Could you check a few things on this drawing? It's one solid part, dimensions in mm from its lowest x, y, z. A direction names the side the tool comes from. Give positions to 0.01 mm unless a question says otherwise; leave off trailing zeros. Loops run counter-clockwise (first coordinate to the right, second up) from the corner with the lowest first, then second, coordinate; pieces in that order, holes last.
1. I need wall thicknesses on line 1 along Y through (x, z) = (6, 24.25); line 2 along X through (y, z) = (3.25, 16.5) (1 decimal); line 3 along Z through (x, y) = (35.5, 8.75). Which ranges of each line are inside material? Lowest first, please.
2. Imagine slicing it at D-D (y = 3.5). List the corners of the cut face in (x, z) for me.
3. For P1, Ø3, axis at x = 9.5, y = 5, coming from the +Z side; P2, Ø1, axis at y = 2, z = 20, coming from the -X side; P3, Ø4, axis at x = 39, z = 14, coming from the -Y side; P4, Ø3, axis at y = 2.5, z = 15.5, coming from the +X side (1 decimal), each with a flat end and sliding along its axis, tell me the tip position at first contact or that it passes through.
4. Imagine slicing it at A-A (z = 6.35). Count the separate pieces of the cut face and the enclosed holes in it.
5. For the marked faces 1, 2 and 3, which set-ups out of +Z, -Z, +X, -X, +Y, -Y let a thin tool reach every point of the face, with its end or its side?
6. Imagine slicing it at C-C (x = 5.5). List the corners of the cut face in (y, z) for me.
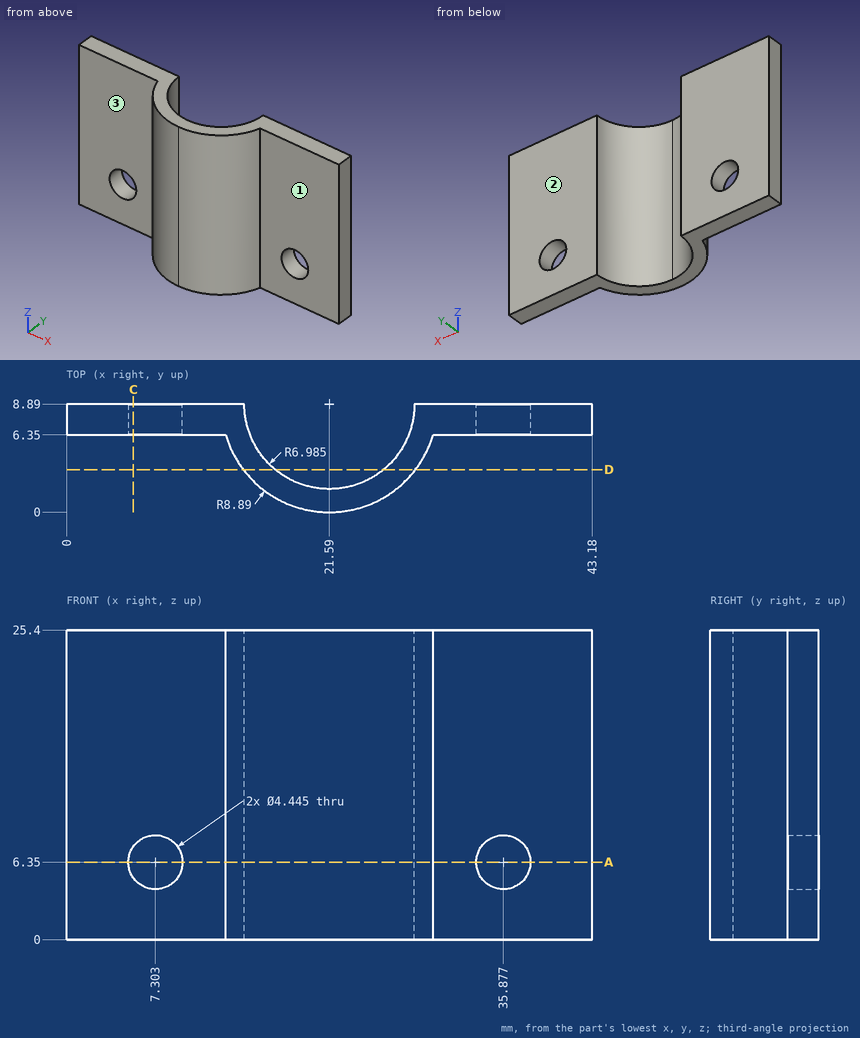
Derived:
1. line 1: y = 6.35 to 8.89
1. line 2: x = 14.7 to 17.5, 25.7 to 28.5
1. line 3: z = 0 to 4.16, 8.54 to 25.4
2. outline: (14.52, 0) - (17.15, 0) - (17.15, 25.4) - (14.52, 25.4) - close; (26.03, 0) - (28.66, 0) - (28.66, 25.4) - (26.03, 25.4) - close
3. P1: stops at z = 25.4
3. P2: stops at x = 15.41
3. P3: stops at y = 6.35
3. P4: stops at x = 29
4. separate pieces: 3
4. enclosed holes: 0
5. face 1: +Z, -Z, +X, -Y
5. face 2: +Z, -Z, +X, -X, +Y
5. face 3: +Z, -Z, -X, -Y
6. outline: (6.35, 0) - (8.89, 0) - (8.89, 5.05) - (6.35, 5.05) - close; (6.35, 7.65) - (8.89, 7.65) - (8.89, 25.4) - (6.35, 25.4) - close
